CAD build for the part. Positions are in the model's coordinates, mm. A direction names the side the tool comes from. Round coordinates to 2 decimals unless told otherwise and drop trailing zeros. Write each loop counter-clockwise with the first axis right and the second up, starting at its lowest first coordinate (ties: lowest second). Pieces come first, ordered by that corner, then holes. Notation, with made-up numbers: (5, 88.5) -> (62, 88.5) arc R11 cw to (62, 101.5) -> close; hole circle Ø5 at (46, 35.5). An arc over 180 degrees is marked (long way). Put each result on its own line as item: value. Start each with the question number.
1. 3-axis set-ups, long thin cutter, end or side, ignore diameter. For faces 1 (the cylindrical face through (16.232, 1.252, 58.176)), 2 (the flat face through (0, -3, 19)): which of +Z, -Z, +X, -X, +Y, -Y reach the whole face in a straight line?
2. Saw through at C-C on y = 1.75. List the corners of the cut face in (x, z), and give its area (3 significant figures).
3. Saw through at A-A on x = 0. List the corners of the cut face in (y, z).
4. Saw through at B-B on x = 5. List the corners of the cut face in (y, z).
5. Flat gauge pins, fed straight in: P1, Ø2, axis at x = 11, z = 9.72, coming from the -Y side; P2, Ø1, axis at x = -5.5, y = 1.5, coming from the -Z side; P3, Ø3.5, axis at x = 0, z = -1.28, coming from the +Y side. Where does each tip first touch, or does it go through?
6. Saw through at D-D on y = -2.25. List the corners of the cut face in (x, z).
7. Drill centre lines: line 1 (Z direction, x = 0, y = 1.25); line 2 (Z direction, x = 0, y = -1.45); line 3 (Y direction, x = -4, z = 37). Where is each one in solid material? Low to high. Write a range as from..to.
8. Pull direction Z, two halves, no side cores. Call faces 3 (the cylindrical face through (12.813, 1.288, 16.703)), 4 (the flat face through (0, 2.54, 37)), 5 (the cylindrical face through (-1.951, -3.626, 0.935)): pulls with the +Z half, pulls with the -Z half, needs draft (parallel to the pull), parting line crosses it, or undercut.
from build123d import *

# Parameters (mm, degrees)
SKETCH1_R           = 1.999999943
SKETCH1_R_2         = 1.1
SKETCH1_R_3         = 8
BOSS_EXTRUDE1_DEPTH = 2.54
FILLET2_R           = 10
SKETCH1_4_R         = 8
SKETCH1_4_R_2       = 1.1
BOSS_EXTRUDE2_DEPTH = 2.999994
SKETCH2_R           = 9
SKETCH2_R_2         = 8
BOSS_EXTRUDE3_DEPTH = 1.27


with BuildPart() as part:
    # Sketch1 → Boss-Extrude1 (new body)
    with BuildSketch(Plane(origin=(0, 0, 0), x_dir=(1, 0, 0), z_dir=(0, 1, 0))):
        with BuildLine():
            Line((20.411129853, -60.145086441), (21.536156884, -59.674942586))
            Line((21.536156884, -59.674942586), (12.379162196, -16.260133485))
            ThreePointArc((12.379162196, -16.260133485), (0, 4.278699998), (-12.379162196, -16.260133485))
            Line((-12.379162196, -16.260133485), (-21.536156884, -59.674942586))
            Line((-21.536156884, -59.674942586), (-20.411129853, -60.145086441))
            ThreePointArc((-20.411129853, -60.145086441), (0, -64.119576268), (20.411129853, -60.145086441))
        make_face()
        with Locations((-16.665975394, -56.223288884)):
            Circle(SKETCH1_R, mode=Mode.SUBTRACT)
        with Locations((16.665975394, -56.223288884)):
            Circle(SKETCH1_R, mode=Mode.SUBTRACT)
        with Locations((-11, -9.721300002)):
            Circle(SKETCH1_R_2, mode=Mode.SUBTRACT)
        with Locations((0, -9.721300002)):
            Circle(SKETCH1_R_3, mode=Mode.SUBTRACT)
        with Locations((0, 1.278699998)):
            Circle(SKETCH1_R_2, mode=Mode.SUBTRACT)
        with Locations((11, -9.721300002)):
            Circle(SKETCH1_R_2, mode=Mode.SUBTRACT)
    extrude(amount=BOSS_EXTRUDE1_DEPTH)

    # Fillet2
    fillet2_edges = [part.edges().sort_by_distance(p)[0] for p in [
        (-12.379162196, 1.27, 16.260133485),
        (12.379162196, 1.27, 16.260133485),
    ]]
    fillet(fillet2_edges, radius=FILLET2_R)

    # Sketch1_4 → Boss-Extrude2 (add)
    with BuildSketch(Plane(origin=(0, 0, 0), x_dir=(1, 0, 0), z_dir=(0, 1, 0))):
        with BuildLine():
            ThreePointArc((-12.379162196, -16.260133485), (0, -23.721300002), (12.379162196, -16.260133485))
            ThreePointArc((12.379162196, -16.260133485), (13.588750324, -13.089662308), (14, -9.721300002))
            ThreePointArc((14, -9.721300002), (-3.368362306, 3.867450323), (-12.379162196, -16.260133485))
        make_face()
        with BuildLine():
            ThreePointArc((-9.9, -9.721300002), (-10.307077747, -10.575617712), (-11.22701591, -10.797619553))
            ThreePointArc((-11.22701591, -10.797619553), (-11.692922253, -8.866982291), (-9.9, -9.721300002))
        make_face(mode=Mode.SUBTRACT)
        with Locations((0, -9.721300002)):
            Circle(SKETCH1_4_R, mode=Mode.SUBTRACT)
        with Locations((0, 1.278699998)):
            Circle(SKETCH1_4_R_2, mode=Mode.SUBTRACT)
        with BuildLine():
            ThreePointArc((12.1, -9.721300002), (11.854317711, -10.414222255), (11.22701591, -10.797619553))
            ThreePointArc((11.22701591, -10.797619553), (10.145682289, -9.028377748), (12.1, -9.721300002))
        make_face(mode=Mode.SUBTRACT)
    extrude(amount=-BOSS_EXTRUDE2_DEPTH)

    # Sketch2 → Boss-Extrude3 (add)
    with BuildSketch(Plane.XZ.offset(2.999994)):
        with Locations((0, 9.721300002)):
            Circle(SKETCH2_R)
        with Locations((0, 9.721300002)):
            Circle(SKETCH2_R_2, mode=Mode.SUBTRACT)
    extrude(amount=BOSS_EXTRUDE3_DEPTH)


solid = part.part
Return value:
1. face 1: +Y, -Y
1. face 2: -Y
2. outline: (-21.54, 59.67) -> (-13.02, 19.28) arc R10 cw to (-13.3, 14.09) arc R14 ccw (long way) to (13.3, 14.09) arc R10 cw to (13.02, 19.28) -> (21.54, 59.67) -> (20.41, 60.15) arc R54.4 ccw to (-20.41, 60.15) -> close; hole circle Ø4 at (-16.67, 56.22); hole circle Ø2.2 at (-11, 9.72); hole circle Ø16 at (0, 9.72); hole circle Ø2.2 at (0, -1.28); hole circle Ø2.2 at (11, 9.72); hole circle Ø4 at (16.67, 56.22)
2. area: 1,850 mm^2
3. outline: (-4.27, 0.72) -> (-3, 0.72) -> (-3, -0.18) -> (2.54, -0.18) -> (2.54, 1.72) -> (-4.27, 1.72) -> close; (-4.27, 17.72) -> (2.54, 17.72) -> (2.54, 64.12) -> (0, 64.12) -> (0, 23.72) -> (-3, 23.72) -> (-3, 18.72) -> (-4.27, 18.72) -> close; (-3, -4.28) -> (2.54, -4.28) -> (2.54, -2.38) -> (-3, -2.38) -> close
4. outline: (-4.27, 2.24) -> (-3, 2.24) -> (-3, -3.36) -> (2.54, -3.36) -> (2.54, 3.48) -> (-4.27, 3.48) -> close; (-4.27, 15.97) -> (2.54, 15.97) -> (2.54, 63.89) -> (0, 63.89) -> (0, 22.8) -> (-3, 22.8) -> (-3, 17.2) -> (-4.27, 17.2) -> close
5. P1: passes through
5. P2: stops at z = -3.36
5. P3: stops at y = 2.54
6. outline: circle Ø28 at (0, 9.72); hole circle Ø2.2 at (-11, 9.72); hole circle Ø16 at (0, 9.72); hole circle Ø2.2 at (0, -1.28); hole circle Ø2.2 at (11, 9.72)
7. line 1: z = -4.28..-2.38, -0.18..1.72, 17.72..64.12
7. line 2: z = -4.28..-2.38, -0.18..1.72, 17.72..23.72
7. line 3: y = 0..2.54
8. face 3: undercut
8. face 4: needs draft
8. face 5: parting line crosses it
